Verification items for the finished model (mm, model axes). Face numbers are marked on the shaded views. A direction names the side the tool comes from. Give positions to 0.01 mm unless a question says otherwise; leave off trailing zeros. Write each loop counter-clockwise with the first axis right and the second up, starting at its lowest first coordinate (ties: lowest second). Pieces come first, ordered by that corner, then holes. Notation, with made-up numbers: (55, 88) -> (113, 88) arc R12 cw to (113, 94) -> close; hole circle Ø10 at (-12, -17). An arc over 180 degrees is marked (long way). Answer as CSV lines item,"result". Start each with the question number.
1) Sectioned sample at C-C on x = 36. Record the cut outline in (y, z), and give its area (3 significant figures).
2) Sectioned sample at B-B on z = 0. Give the number of separate pieces and of enclosed holes in the cut face, and give its area (3 significant figures).
3) Mould release check, pull along X, two halves, no side actions. Record for the marked faces 1, 2, 3 and 4: released by +X, released by -X, zero draft, split by the parting line, or undercut.
4) Sectioned sample at A-A on x = 0. Record the cut outline in (y, z), and give its area (3 significant figures).
5) Material ranges on L1, parallel to X at y = 60.5, z = -5.5; L2, parallel to X at y = 6.5, z = 0; L3, parallel to Y at x = 17.5, z = -6.5, recorded low to high.
6) Tool access check on the marked faces 5 and 6. Record the directions out of +Z, -Z, +X, -X, +Y, -Y that give a thin tool (end or side, any length) a straight path to the whole face; none if there is none.
7) Gauge pin test, flat ends, axial feed: pin 1 Ø1 at (x, z) = (-15.5, -4) entering from +Y; pin 2 Ø6 at (x, z) = (-51.5, 1) entering from +Y (3 decimals). Record the tip position at first contact, or that the pin passes through.
8) Sectioned sample at D-D on x = -41.5. Record the cut outline in (y, z).
```python
from build123d import *

# Parameters (mm, degrees)
SKETCH1_R           = 2.5
BOSS_EXTRUDE1_DEPTH = 70
CUT_EXTRUDE1_START  = -10
SKETCH2_W           = 120
SKETCH2_H           = 40
CUT_EXTRUDE1_DEPTH  = 110
SKETCH3_R           = 1.3
SKETCH3_R_2         = 5
CUT_EXTRUDE2_DEPTH  = 10
FILLET1_R           = 5
FILLET2_R           = 20


with BuildPart() as part:
    # Sketch1 → Boss-Extrude1 (new, symmetric)
    with BuildSketch(Plane(origin=(0, 0, 0), x_dir=(0, 0, -1), z_dir=(1, 0, 0))):
        with BuildLine():
            Line((-20, 0), (20, 0))
            Line((20, 0), (20, 10))
            Line((20, 10), (10, 100))
            ThreePointArc((10, 100), (0, 110), (-10, 100))
            Line((-10, 100), (-20, 10))
            Line((-20, 10), (-20, 0))
        make_face()
        with Locations((0, 100)):
            Circle(SKETCH1_R, mode=Mode.SUBTRACT)
    extrude(amount=BOSS_EXTRUDE1_DEPTH, both=True)

    # Sketch2 → Cut-Extrude1 (cut)
    with BuildSketch(Plane.XZ.offset(CUT_EXTRUDE1_START)):
        Rectangle(SKETCH2_W, SKETCH2_H)
    extrude(amount=-CUT_EXTRUDE1_DEPTH, mode=Mode.SUBTRACT)

    # Sketch3 → Cut-Extrude2 (cut)
    with BuildSketch(Plane.XZ):
        with Locations(Location((-4, 15.491933385, 0), (0, 0, 270))):
            Circle(SKETCH3_R)
        with Locations(Location((15.416407865, -4.281865077, 0), (0, 0, 270))):
            Circle(SKETCH3_R)
        with Locations(Location((-11.416407865, -11.210068308, 0), (0, 0, 270))):
            Circle(SKETCH3_R)
        with Locations(Location((0, 0, 0), (0, 0, 270))):
            Circle(SKETCH3_R_2)
    extrude(amount=-CUT_EXTRUDE2_DEPTH, mode=Mode.SUBTRACT)

    # Fillet1
    fillet1_edges = [part.edges().sort_by_distance(p)[0] for p in [
        (70, 5, -20),
        (70, 55, -15),
        (70, 110, 0),
        (70, 55, 15),
        (70, 5, 20),
        (-70, 55, 15),
        (-70, 110, 0),
        (-70, 55, -15),
        (-70, 5, -20),
        (-70, 5, 20),
    ]]
    fillet(fillet1_edges, radius=FILLET1_R)

    # Fillet2
    fillet2_edges = [part.edges().sort_by_distance(p)[0] for p in [
        (-60, 10, 0),
        (60, 10, 0),
    ]]
    fillet(fillet2_edges, radius=FILLET2_R)


solid = part.part
```
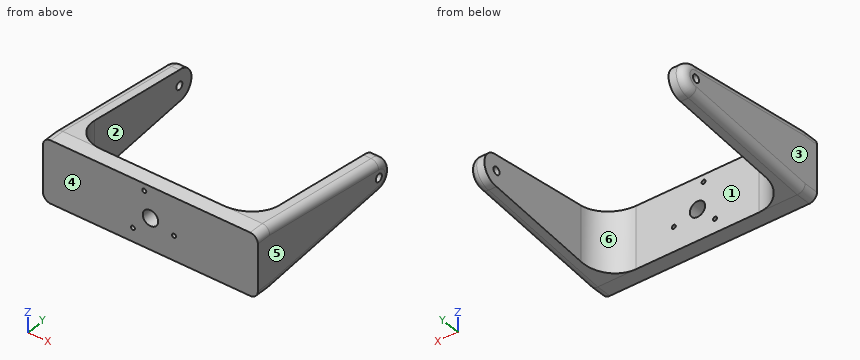
Ans:
1,outline,"(0, -20) -> (10, -20) -> (10, 20) -> (0, 20) -> close"
1,area,"400 mm²"
2,separate pieces,"4"
2,enclosed holes,"0"
2,area,"3,360 mm²"
3,face 1,"undercut"
3,face 2,"undercut"
3,face 3,"released by -X"
3,face 4,"zero draft"
4,outline,"(0, -20) -> (10, -20) -> (10, -5) -> (0, -5) -> close; (0, 5) -> (10, 5) -> (10, 20) -> (0, 20) -> close"
4,area,"300 mm²"
5,L1,"x = -70 to -60, 60 to 70"
5,L2,"x = -70 to -5, 5 to 70"
5,L3,"y = 0 to 10"
6,face 5,"+Z, -Z, +X, +Y, -Y"
6,face 6,"+Z, -Z, +Y"
7,pin 1,"stops at y = 10"
7,pin 2,"stops at y = 16.225"
8,outline,"(0, -20) -> (10, -20) -> (10.06, -19.99) -> (10.06, 19.99) -> (10, 20) -> (0, 20) -> close"
